Verification items for the finished model (mm, model axes). A direction names the side the tool comes from. Give positions to 0.01 mm unless a question says otherwise; leave off trailing zeros. Loops run counter-clockwise (first coordinate to the right, second up) from the corner with the lowest first, then second, coordinate; pieces in that order, holes last. Notation, with made-up numbers: M 74.25,3.5 L 107.25,3.5 A37 cw 107.25,41.5 Z; hole C 85,27.5 d2. An arc over 180 degrees is marked long. Use CSV: the item, a comma, the result in double quotes.
from build123d import *

# Parameters (mm, degrees)
F0_R          = 50.8
F1_DEPTH      = 330.2
F1_DEPTH_BACK = 508
F3_W          = 177.8
F3_H          = 177.8
F4_DEPTH      = 177.8
F6_START      = -1.27
F5_W          = 170.18
F5_H          = 170.18
F6_DEPTH      = 175.006
F2_R          = 47.625
F7_DEPTH      = 914.4


with BuildPart() as f1:
    # F0 (on Front) → F1 (new body, two sides)
    with BuildSketch(Plane.XZ) as f1_sk:
        Circle(F0_R)
    extrude(amount=F1_DEPTH)
    extrude(f1_sk.sketch, amount=-F1_DEPTH_BACK)

    # F3 (on Front) → F4 (join)
    with BuildSketch(Plane.XZ):
        Rectangle(F3_W, F3_H)
    extrude(amount=-F4_DEPTH)

    # F5 (on face) → F6 (cut)
    with BuildSketch(Plane(origin=(0, 177.8, 0), x_dir=(-1, 0, 0), z_dir=(0, 1, 0)).offset(F6_START)):
        Rectangle(F5_W, F5_H)
    extrude(amount=-F6_DEPTH, mode=Mode.SUBTRACT)

    # F2 (on face) → F7 (cut)
    with BuildSketch(Plane.XZ.offset(330.2)):
        Circle(F2_R)
    extrude(amount=-F7_DEPTH, mode=Mode.SUBTRACT)


solid = f1.part
(1) Section check B-B on z = 0. Record the cut outline in (x, y) (3 decimals).
Calculated:
outline,"M -88.9,0 L -50.8,0 L -50.8,-330.2 L -47.625,-330.2 L -47.625,1.524 L -85.09,1.524 L -85.09,176.53 L -47.625,176.53 L -47.625,508 L -50.8,508 L -50.8,177.8 L -88.9,177.8 Z; M 47.625,-330.2 L 50.8,-330.2 L 50.8,0 L 88.9,0 L 88.9,177.8 L 50.8,177.8 L 50.8,508 L 47.625,508 L 47.625,176.53 L 85.09,176.53 L 85.09,1.524 L 47.625,1.524 Z"
(2) Scan lines: L1, parallel to Z at x = -3.5, y = 173; L2, parallel to Y at x = -33, z = 77. Record each from-to range of solid material in increasing order. Write a range as from..to.
Calculated:
L1,"z = -88.9..-85.09, 85.09..88.9"
L2,"y = 0..1.52, 176.53..177.8"
(3) Section check D-D on z = -75. Record the cut outline in (x, y).
Calculated:
outline,"M -88.9,0 L 88.9,0 L 88.9,177.8 L -88.9,177.8 Z; hole M -85.09,1.52 L 85.09,1.52 L 85.09,176.53 L -85.09,176.53 Z"
(4) Tool access check on faces 5 (the flat face through (1, 90, -85.09)), 6 (the flat face through (-1, 88, 88.9)), 7 (the cylindrical face through (-11.012, 340.589, -49.592)), 8 (the flat face through (38, 0, 41)). Record the directions out of +Z, -Z, +X, -X, +Y, -Y that give a thin tool (end or side, any length) a straight path to the whole face; none if there is none.
Calculated:
face 5,"none"
face 6,"+Z, +X, -X, +Y, -Y"
face 7,"+Y"
face 8,"-Y"
(5) Depth check by flat-ended pin: pin 1 Ø1 at (x, y) = (35.5, 253) entering from +Z; pin 2 Ø3 at (x, y) = (2, 357.5) entering from -Z; pin 3 Ø2 at (y, z) = (-14.5, -46) entering from +X. Enter the tip coordinate at first touch or a pass-through.
Calculated:
pin 1,"stops at z = 36.82"
pin 2,"stops at z = -50.8"
pin 3,"stops at x = 23.57"
(6) Section check C-C on y = 92. Record the cut outline in (x, z).
Calculated:
outline,"M -88.9,-88.9 L 88.9,-88.9 L 88.9,88.9 L -88.9,88.9 Z; hole M -85.09,-85.09 L 85.09,-85.09 L 85.09,85.09 L -85.09,85.09 Z"
(7) Mould release check, pull along X, two halves, no side actions. Record for faces 1 (the flat face through (-15.3, 508, 45.4)), 2 (the cylindrical face through (-11.012, -167.411, -49.592)), 3 (the flat face through (-88.9, 88, -1)), 4 (the cylindrical face through (-37.794, 339.945, -28.979)): released by +X, released by -X, zero draft, split by the parting line, or undercut.
Calculated:
face 1,"zero draft"
face 2,"split by the parting line"
face 3,"released by -X"
face 4,"undercut"
(8) Section check A-A on x = 0. Record the cut outline in (y, z) (3 decimals).
Calculated:
outline,"M -330.2,-50.8 L 0,-50.8 L 0,-88.9 L 177.8,-88.9 L 177.8,-50.8 L 508,-50.8 L 508,-47.625 L 176.53,-47.625 L 176.53,-85.09 L 1.524,-85.09 L 1.524,-47.625 L -330.2,-47.625 Z; M -330.2,47.625 L 1.524,47.625 L 1.524,85.09 L 176.53,85.09 L 176.53,47.625 L 508,47.625 L 508,50.8 L 177.8,50.8 L 177.8,88.9 L 0,88.9 L 0,50.8 L -330.2,50.8 Z"
